Build history of the part. All positions in model axes, mm. Give positions to 0.01 mm unless a question says otherwise; leave off trailing zeros. Loops run counter-clockwise (first coordinate to the right, second up) from the corner with the lowest first, then second, coordinate; pieces in that order, holes last.
1) Band-saw the part on D-D on y = 2.35. State how many separate pieces and enclosed holes the cut face has, then the cut area to 3 significant figures.
2) Wall check: line 1 (Z direction, x = 0, y = 1.95); line 2 (X direction, y = 0.7, z = -5); line 3 (Z direction, x = 25, y = 0.95). Give the ranges that are in metal, low to high.
3) Flat gauge pins, fed straight in: P1, Ø2.5, axis at x = 0, z = 5, coming from the -Y side; P2, Ø1.6, axis at x = -27, y = 1.5, coming from the +Z side; P3, Ø1.6, axis at x = -27.5, y = 2.5, coming from the -Z side. Where does each tip first touch, or does it go through?
4) Band-saw the part on C-C on z = 1. List the corners of the cut face in (x, y), then the cut area to 3 significant figures.
5) Band-saw the part on B-B on x = 5.5. List the corners of the cut face in (y, z).
6) Band-saw the part on A-A on x = -40. List the corners of the cut face in (y, z), then the cut area to 3 significant figures.
```python
from build123d import *

# Parameters (mm, degrees)
SKETCH1_R           = 1.5025
SKETCH1_W           = 42
SKETCH1_H           = 21
BOSS_EXTRUDE1_DEPTH = 3.25


with BuildPart() as part:
    # Sketch1 → Boss-Extrude1 (new body)
    with BuildSketch(Plane(origin=(0, 0, 0), x_dir=(1, 0, 0), z_dir=(0, 1, 0))):
        with BuildLine():
            Line((-49.5, 18.5), (-35.5, 18.5))
            Line((-35.5, 18.5), (-30.5, 13.5))
            Line((-30.5, 13.5), (-24.5, 13.5))
            Line((-24.5, 13.5), (-19.5, 18.5))
            Line((-19.5, 18.5), (49.5, 18.5))
            ThreePointArc((49.5, 18.5), (52.328427125, 17.328427125), (53.5, 14.5))
            Line((53.5, 14.5), (53.5, -14.5))
            ThreePointArc((53.5, -14.5), (52.328427125, -17.328427125), (49.5, -18.5))
            Line((49.5, -18.5), (-19.5, -18.5))
            Line((-19.5, -18.5), (-24.5, -13.5))
            Line((-24.5, -13.5), (-30.5, -13.5))
            Line((-30.5, -13.5), (-35.5, -18.5))
            Line((-35.5, -18.5), (-49.5, -18.5))
            ThreePointArc((-49.5, -18.5), (-52.328427125, -17.328427125), (-53.5, -14.5))
            Line((-53.5, -14.5), (-53.5, 14.5))
            ThreePointArc((-53.5, 14.5), (-52.328427125, 17.328427125), (-49.5, 18.5))
        make_face()
        with Locations((25, -15)):
            Circle(SKETCH1_R, mode=Mode.SUBTRACT)
        with Locations((-40, -10)):
            Circle(SKETCH1_R, mode=Mode.SUBTRACT)
        with Locations((-30, -10)):
            Circle(SKETCH1_R, mode=Mode.SUBTRACT)
        with Locations((0, -5)):
            Circle(SKETCH1_R, mode=Mode.SUBTRACT)
        with Locations((50, -5)):
            Circle(SKETCH1_R, mode=Mode.SUBTRACT)
        with Locations((0, 5)):
            Circle(SKETCH1_R, mode=Mode.SUBTRACT)
        with Locations((50, 5)):
            Circle(SKETCH1_R, mode=Mode.SUBTRACT)
        with Locations((-40, 10)):
            Circle(SKETCH1_R, mode=Mode.SUBTRACT)
        with Locations((-30, 10)):
            Circle(SKETCH1_R, mode=Mode.SUBTRACT)
        with Locations((25, 15)):
            Circle(SKETCH1_R, mode=Mode.SUBTRACT)
        with Locations((-50, -10)):
            Circle(SKETCH1_R, mode=Mode.SUBTRACT)
        with Locations((-50, 10)):
            Circle(SKETCH1_R, mode=Mode.SUBTRACT)
        with Locations((24.5, 0)):
            Rectangle(SKETCH1_W, SKETCH1_H, mode=Mode.SUBTRACT)
    extrude(amount=BOSS_EXTRUDE1_DEPTH)


solid = part.part
```
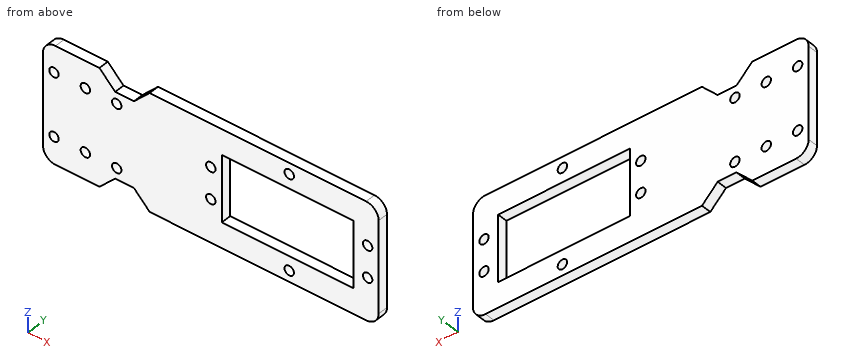
Findings below:
1. separate pieces: 1
1. enclosed holes: 13
1. area: 2,870 mm2
2. line 1: z = -18.5 to -6.5, -3.5 to 3.5, 6.5 to 18.5
2. line 2: x = -53.5 to -1.5, 1.5 to 3.5, 45.5 to 48.5, 51.5 to 53.5
2. line 3: z = -18.5 to -16.5, -13.5 to -10.5, 10.5 to 13.5, 16.5 to 18.5
3. P1: passes through
3. P2: stops at z = 13.5
3. P3: stops at z = -13.5
4. outline: (-53.5, 0) - (3.5, 0) - (3.5, 3.25) - (-53.5, 3.25) - close; (45.5, 0) - (53.5, 0) - (53.5, 3.25) - (45.5, 3.25) - close
4. area: 211 mm2
5. outline: (0, -18.5) - (3.25, -18.5) - (3.25, -10.5) - (0, -10.5) - close; (0, 10.5) - (3.25, 10.5) - (3.25, 18.5) - (0, 18.5) - close
6. outline: (0, -18.5) - (3.25, -18.5) - (3.25, -11.5) - (0, -11.5) - close; (0, -8.5) - (3.25, -8.5) - (3.25, 8.5) - (0, 8.5) - close; (0, 11.5) - (3.25, 11.5) - (3.25, 18.5) - (0, 18.5) - close
6. area: 101 mm2
